Can you work these out from the model? Positions are in its coordinate system, mm. Face numbers are marked on the shaded views. A direction names the side the tool comes from. Round coordinates to 2 decimals unless told otherwise and drop trailing zeros. Write each loop counter-clockwise with the first axis right and the second up, starting at its lowest first coordinate (ties: lowest second). Pieces come first, ordered by that corner, then holes. Notation, with made-up numbers: (88.5, 45) - (118.5, 45) arc R20 ccw to (118.5, 75) - close; hole circle Ø4 at (3.25, -32). An arc over 180 degrees is marked (long way). One line per item, written item: value. Start each with the question number.
(1) I want a section at A-A on x = 0.3. List the corners of the cut face in (y, z) for me (3 decimals).
(2) I want a section at B-B on z = -2. List the corners of the cut face in (x, y) for me (3 decimals).
(3) If I drill on L1, parallel to Y at x = 1.9, z = 2.75 (3 decimals); L2, parallel to X at y = -0.7, z = 3.5; L3, parallel to Z at x = 0.3, y = 0.65, over which ranges is the centre line in solid material (lowest first)? Write a range as from..to.
(4) On a 3-axis mill with a long thin cutter (end or side, diameter ignored), from which of +Z, -Z, +X, -X, +Y, -Y can I reach the whole of each face in a straight line? I mean the marked faces 1 and 2. Say none if no direction works.
from build123d import *

# Parameters (mm, degrees)
CROQUIS1_W              = 7.5
CROQUIS1_H              = 1.87
SALIENTE_EXTRUIR1_DEPTH = 3
CORTAR_EXTRUIR1_REACH   = 10.132
CROQUIS2_W              = 2
CROQUIS2_H              = 0.35
REDONDEO1_R             = 0.5


with BuildPart() as part:
    # Croquis1 → Saliente-Extruir1 (new body)
    with BuildSketch(Plane(origin=(0, 0, 0), x_dir=(0, 0, -1), z_dir=(1, 0, 0))):
        Rectangle(CROQUIS1_W, CROQUIS1_H)
    extrude(amount=SALIENTE_EXTRUIR1_DEPTH)

    # Croquis2 → Cortar-Extruir1 (cut, up to next)
    with BuildSketch(Plane.XY.offset(3.75), mode=Mode.PRIVATE) as cortar_extruir1_sk1:
        with Locations((1, -0.76)):
            Rectangle(CROQUIS2_W, CROQUIS2_H)
    cortar_extruir1_tool1 = extrude(cortar_extruir1_sk1.sketch, amount=-CORTAR_EXTRUIR1_REACH, mode=Mode.PRIVATE) & part.part
    add(cortar_extruir1_tool1.solids().sort_by_distance((1, -0.76, 3.75))[0], mode=Mode.SUBTRACT)

    # Redondeo1
    redondeo1_edges = [part.edges().sort_by_distance(p)[0] for p in [
        (1.5, 0.935, 3.75),
        (1.5, 0.935, -3.75),
    ]]
    fillet(redondeo1_edges, radius=REDONDEO1_R)


solid = part.part
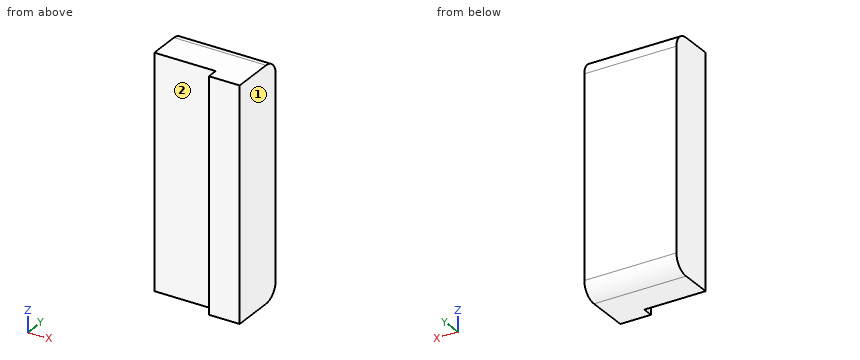
Established:
1. outline: (-0.585, -3.75) - (0.435, -3.75) arc R0.5 ccw to (0.935, -3.25) - (0.935, 3.25) arc R0.5 ccw to (0.435, 3.75) - (-0.585, 3.75) - close
2. outline: (0, -0.585) - (2, -0.585) - (2, -0.935) - (3, -0.935) - (3, 0.935) - (0, 0.935) - close
3. L1: -0.585..0.935
3. L2: 2..3
3. L3: -3.7..3.7
4. face 1: +Z, -Z, +X, +Y, -Y
4. face 2: +Z, -Z, -X, -Y
